from build123d import *

# Parameters (mm, degrees)
F1_DEPTH = 1.5


with BuildPart() as f1:
    # F0 (on Front) → F1 (new body)
    with BuildSketch(Plane.XZ):
        with BuildLine():
            Line((9, -19), (15, -19))
            Line((15, -19), (15, -17.5))
            Line((15, -17.5), (18, -17.5))
            Line((18, -17.5), (18, 16.5))
            Line((18, 16.5), (15, 16.5))
            Line((15, 16.5), (15, 18))
            Line((15, 18), (9, 18))
            Line((9, 18), (9, 16.5))
            Line((9, 16.5), (-10, 16.5))
            Line((-10, 16.5), (-10, 18))
            Line((-10, 18), (-16, 18))
            Line((-16, 18), (-16, 16.5))
            Line((-16, 16.5), (-19.5, 16.5))
            Line((-19.5, 16.5), (-19.5, 15.634314))
            ThreePointArc((-19.5, 15.634314), (-19.306113, 14.57331), (-18.749514, 13.649449))
            Line((-18.749514, 13.649449), (-11.157439, 5.045098))
            ThreePointArc((-11.157439, 5.045098), (-10.417146, 3.307324), (-10.862109, 1.471595))
            ThreePointArc((-10.862109, 1.471595), (-11.709917, -0.434306), (-12, -2.5))
            ThreePointArc((-12, -2.5), (-11.861475, -3.93481), (-11.451019, -5.316619))
            ThreePointArc((-11.451019, -5.316619), (-11.32884, -7.20155), (-12.357341, -8.785873))
            Line((-12.357341, -8.785873), (-18.374085, -13.599268))
            ThreePointArc((-18.374085, -13.599268), (-19.20391, -14.642308), (-19.5, -15.941875))
            Line((-19.5, -15.941875), (-19.5, -17.5))
            Line((-19.5, -17.5), (-16, -17.5))
            Line((-16, -17.5), (-16, -19))
            Line((-16, -19), (-10, -19))
            Line((-10, -19), (-10, -17.5))
            Line((-10, -17.5), (9, -17.5))
            Line((9, -17.5), (9, -19))
        make_face()
        with BuildLine():
            ThreePointArc((-2.5, -2.5), (-4.5, -4.5), (-6.5, -2.5))
            ThreePointArc((-6.5, -2.5), (-4.5, -0.5), (-2.5, -2.5))
        make_face(mode=Mode.SUBTRACT)
        with BuildLine():
            ThreePointArc((10.470654, -8.054456), (7.629322, -8.385303), (7.361973, -5.537295))
            ThreePointArc((7.361973, -5.537295), (8.634848, 5.219866), (-0.526307, 11))
            ThreePointArc((-0.526307, 11), (-2.526307, 13), (-0.526307, 15))
            ThreePointArc((-0.526307, 15), (12.245156, 6.94198), (10.470654, -8.054456))
        make_face(mode=Mode.SUBTRACT)
    extrude(amount=F1_DEPTH)


solid = f1.part
Build history of the part. All positions in model axes, mm. A direction names the side the tool comes from. Give positions to 0.01 mm unless a question says otherwise; leave off trailing zeros. Order: outer loops, then holes, each group sorted by start corner. A loop starts at its lowest first (then second) coordinate and runs counter-clockwise, first axis right, second up. Notation, with made-up numbers: M 84.25,36 L 98.25,36 A29 ccw 98.25,64 Z; hole C 20,47.25 d8. An arc over 180 degrees is marked long. Use one line per item in the form item = value.
Q1. Which spindle directions (+Z, -Z, +X, -X, +Y, -Y) get a long thin tool onto all of the face, cutting with end or side? Do faces 5 (the flat face through (17, -1, 16.5)), 6 (the cylindrical face through (-11.865, -0.74, -3.915)), 7 (the flat face through (9, -1, -18)), 8 (the flat face through (16, -1, -17.5)), 9 (the flat face through (-16, -1, 17)). Say none if no direction does.
Conclusion:
face_5 = +Z, +X, +Y, -Y
face_6 = -X, +Y, -Y
face_7 = -Z, +Y, -Y
face_8 = -Z, +X, +Y, -Y
face_9 = +Z, -X, +Y, -Y
Q2. Slice it at D-D, the plane z = -10. Write the cut outline in (x, y) (3 decimals), and give its area (3 significant figures).
Conclusion:
outline = M -13.875,-1.5 L 18,-1.5 L 18,0 L -13.875,0 Z
area = 47.8 mm2
Q3. Wall check: probe 1 along Z at (x, y) = (-4.5, -0.4); probe 2 along Z at (x, y) = (-9, -1.25); probe 3 along Z at (x, y) = (1, -0.9). Give the ranges that are in metal, low to high.
Conclusion:
probe_1 = -17.5 to -4.5, -0.5 to 16.5
probe_2 = -17.5 to 16.5
probe_3 = -17.5 to 10.88, 14.92 to 16.5
Q4. Slice it at A-A, the plane x = -4.5. Write the cut outline in (y, z).
Conclusion:
outline = M -1.5,-17.5 L 0,-17.5 L 0,-4.5 L -1.5,-4.5 Z; M -1.5,-0.5 L 0,-0.5 L 0,16.5 L -1.5,16.5 Z
Q5. Pull direction X, two halves, no side cores. Call faces 1 (the cylindrical face through (-11.7, -0.7, -0.4)), 2 (the flat face through (18, -1, -1)), 3 (the flat face through (-13, -1, 18)), 4 (the flat face through (9, -1, 17)): released by +X, released by -X, zero draft, split by the parting line, or undercut.
Conclusion:
face_1 = released by -X
face_2 = released by +X
face_3 = zero draft
face_4 = undercut
Q6. Slice it at C-C, the plane y = -0.8. State how many separate pieces and enclosed holes the cut face has, and give its area (3 significant figures).
Conclusion:
separate_pieces = 1
enclosed_holes = 2
area = 1,000 mm2
Q7. Slice it at B-B, the plane z = 10. Write the cut outline in (x, y).
Conclusion:
outline = M -15.53,-1.5 L 3.87,-1.5 L 3.87,0 L -15.53,0 Z; M 10.27,-1.5 L 18,-1.5 L 18,0 L 10.27,0 Z
Q8. Pin check, flat tips, straight feed: P1, Ø4, axis at x = -5.5, z = 13, coming from the +Y side; P2, Ø0.8, axis at y = -1, z = -18, coming from the +X side; P3, Ø0.8, axis at x = -17.5, y = -0.5, coming from the +Z side. Stop position of each tip, or through.
Conclusion:
P1 = 0
P2 = 15
P3 = 16.5
